```python
from build123d import *

# Parameters (mm, degrees)
F0_W      = 18.4
F0_H      = 14.3
F1_DEPTH  = 5
F2_W      = 18.4
F2_H      = 14.3
F3_DEPTH  = 15
F4_W      = 21
F4_H      = 18
F5_DEPTH  = 2
F6_W      = 8
F6_H      = 2.9
F6_H_2    = 5.2
F7_DEPTH  = 3
F8_W      = 2
F8_H      = 11.251825
F9_DEPTH  = 3
F11_DEPTH = 5
F12_W     = 3
F12_H     = 2
F13_DEPTH = 5


with BuildPart() as f1:
    # F0 (on Top) → F1 (new body)
    with BuildSketch(Plane.XY):
        Polygon((-10, 24), (-22.5, 24), (-22.5, 0), (22.2, 0), (22.2, 24), (10, 24), (10, 18), (-10, 18), align=None)
        with Locations((0, 9.15)):
            Rectangle(F0_W, F0_H, mode=Mode.SUBTRACT)
        with BuildLine():
            Line((-18.4, 6), (-18.4, 19))
            ThreePointArc((-18.4, 19), (-16.5, 20.9), (-14.6, 19))
            Line((-14.6, 19), (-14.6, 6))
            ThreePointArc((-14.6, 6), (-16.5, 4.1), (-18.4, 6))
        make_face(mode=Mode.SUBTRACT)
        with BuildLine():
            Line((14.3, 6), (14.3, 19))
            ThreePointArc((14.3, 19), (16.2, 20.9), (18.1, 19))
            Line((18.1, 19), (18.1, 6))
            ThreePointArc((18.1, 6), (16.2, 4.1), (14.3, 6))
        make_face(mode=Mode.SUBTRACT)
    extrude(amount=F1_DEPTH)

    # F2 (on face) → F3 (join)
    with BuildSketch(Plane.XY.offset(5)):
        Polygon((-10.65, 18), (-10.65, 0), (10.35, 0), (10.35, 18), (10, 18), (-10, 18), align=None)
        with Locations((0, 9.15)):
            Rectangle(F2_W, F2_H, mode=Mode.SUBTRACT)
    extrude(amount=F3_DEPTH)

    # F4 (on face) → F5 (join)
    with BuildSketch(Plane.XY.offset(20)):
        with Locations((-0.15, 9)):
            Rectangle(F4_W, F4_H)
    extrude(amount=F5_DEPTH)

    # F6 (on face) → F7 (cut)
    with BuildSketch(Plane.XZ):
        with Locations((-5, 18.55)):
            Rectangle(F6_W, F6_H)
        with Locations((4.85, 18.55)):
            Rectangle(F6_W, F6_H)
        with Locations((-5, 12.4)):
            Rectangle(F6_W, F6_H_2)
        with Locations((4.85, 12.4)):
            Rectangle(F6_W, F6_H_2)
        with Locations((-5, 5.05)):
            Rectangle(F6_W, F6_H)
        with Locations((4.85, 5.05)):
            Rectangle(F6_W, F6_H)
    extrude(amount=-F7_DEPTH, mode=Mode.SUBTRACT)

    # F8 (on face) → F9 (cut)
    with BuildSketch(Plane(origin=(0, 18, 0), x_dir=(-1, 0, 0), z_dir=(0, 1, 0))):
        with Locations((-3.5, 3.374087)):
            Rectangle(F8_W, F8_H)
        with Locations((3.5, 3.374087)):
            Rectangle(F8_W, F8_H)
    extrude(amount=-F9_DEPTH, mode=Mode.SUBTRACT)

    # F10 (on face) → F11 (join)
    with BuildSketch(Plane.YZ.offset(2.5)):
        Polygon((16.3, 0), (16.3, 3), (15.3, 3), align=None)
    extrude(amount=-F11_DEPTH)

    # F12 (on face) → F13 (cut)
    with BuildSketch(Plane.XY.offset(22)):
        with Locations((-0.15, 14)):
            Rectangle(F12_W, F12_H)
    extrude(amount=-F13_DEPTH, mode=Mode.SUBTRACT)


solid = f1.part
```
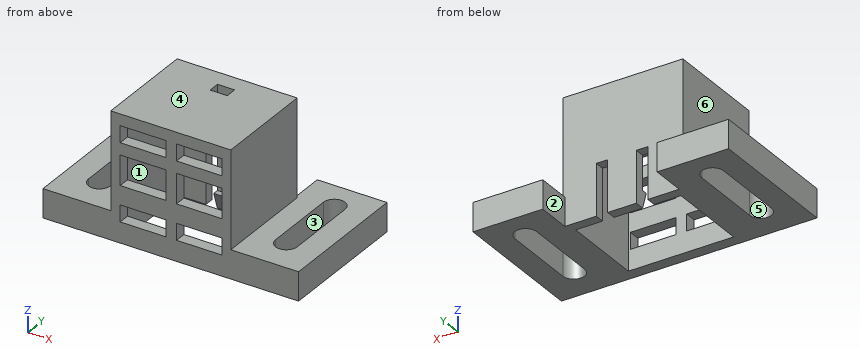
Input: part model. Units: mm. Frame: model coordinates. Face numbers are marked on the shaded views. A direction names the side the tool comes from. Coordinates: 2 decimals unless noted, no trailing zeros. Write each loop counter-clockwise with the first axis right and the second up, starting at its lowest first coordinate (ties: lowest second). Pieces come first, ordered by that corner, then holes. Notation, with made-up numbers: (-0.75, -23) -> (34.25, -23) arc R12 ccw to (34.25, -17) -> close; hole circle Ø8 at (-34.75, 1.25). An arc over 180 degrees is marked (long way). Answer as a JSON object with one key per item and string values.
1. Access query for the marked faces 1, 2 and 3. Directions: +Z, -Z, +X, -X, +Y, -Y. A direction counts if a zero-diameter tool reaches every point of the face in a straight line with its end or side. Return the directions, or none.
Result set:
{"face 1": "-Z", "face 2": "+Z, -Z, +Y", "face 3": "+Z, -Z"}
2. Section A-A on y = 16.75. Return the cut outline in (x, z).
Result set:
{"outline": "(-22.5, 0) -> (-18.4, 0) -> (-18.4, 5) -> (-22.5, 5) -> close; (-14.6, 0) -> (-4.5, 0) -> (-4.5, 9) -> (-2.5, 9) -> (-2.5, 0) -> (2.5, 0) -> (2.5, 9) -> (4.5, 9) -> (4.5, 0) -> (14.3, 0) -> (14.3, 5) -> (10.35, 5) -> (10.35, 22) -> (-10.65, 22) -> (-10.65, 5) -> (-14.6, 5) -> close; (18.1, 0) -> (22.2, 0) -> (22.2, 5) -> (18.1, 5) -> close"}
3. Mould query, pull axis X, two halves, no side actions, for the marked faces 4, 5 and 6. Classes: released by +X, released by -X, zero draft, split by the parting line, or undercut.
Result set:
{"face 4": "zero draft", "face 5": "undercut", "face 6": "released by -X"}
4. Section D-D on z = 5.5. Return the cut outline in (x, y), then the cut area to 3 significant figures.
Result set:
{"outline": "(-10.65, 0) -> (-9, 0) -> (-9, 2) -> (-9.2, 2) -> (-9.2, 16.3) -> (-4.5, 16.3) -> (-4.5, 18) -> (-10.65, 18) -> close; (-2.5, 16.3) -> (2.5, 16.3) -> (2.5, 18) -> (-2.5, 18) -> close; (-1, 0) -> (0.85, 0) -> (0.85, 2) -> (-1, 2) -> close; (4.5, 16.3) -> (9.2, 16.3) -> (9.2, 2) -> (8.85, 2) -> (8.85, 0) -> (10.35, 0) -> (10.35, 18) -> (4.5, 18) -> close", "area": "76.1 mm2"}
5. Section B-B on z = 19.5. Return the cut outline in (x, y).
Result set:
{"outline": "(-10.65, 0) -> (-9, 0) -> (-9, 2) -> (-9.2, 2) -> (-9.2, 16.3) -> (9.2, 16.3) -> (9.2, 2) -> (8.85, 2) -> (8.85, 0) -> (10.35, 0) -> (10.35, 18) -> (-10.65, 18) -> close; (-1, 0) -> (0.85, 0) -> (0.85, 2) -> (-1, 2) -> close"}
6. Section C-C on x = 7. Return the cut outline in (y, z).
Result set:
{"outline": "(0, 0) -> (2, 0) -> (2, 3.6) -> (0, 3.6) -> close; (0, 6.5) -> (2, 6.5) -> (2, 9.8) -> (0, 9.8) -> close; (0, 15) -> (2, 15) -> (2, 17.1) -> (0, 17.1) -> close; (0, 20) -> (16.3, 20) -> (16.3, 0) -> (18, 0) -> (18, 22) -> (0, 22) -> close"}
7. Material intervals for line 1 (X direction, y = 12, z = 4); line 2 (X direction, y = 8.5, z = 14.5); line 3 (Z direction, x = -14.5, y = 19.25), sorted ascending. Write a range as from..to.
Result set:
{"line 1": "x = -22.5..-18.4, -14.6..-9.2, 9.2..14.3, 18.1..22.2", "line 2": "x = -10.65..-9.2, 9.2..10.35", "line 3": "z = 0..5"}
8. First-contact query: P1, Ø0.6, axis at y = 13.5, z = 21, coming from the -X side; P2, Ø1.6, axis at x = 0.5, z = 21.5, coming from the +Y side; P3, Ø1.6, axis at y = 14, z = 20.5, coming from the +X side; P4, Ø10, axis at x = 16.5, z = 16.5, coming from the -Y side. Flat tips, straight axial feed; report the tip coordinate or a pass-through.
Result set:
{"P1": "stops at x = -10.65", "P2": "stops at y = 18", "P3": "stops at x = 10.35", "P4": "passes through"}
